```python
from build123d import *

# Parameters (mm, degrees)
F0_W        = 50
F0_H        = 30
F1_DEPTH    = 15
F2_SIZE2    = 12
F2_SIZE     = 40
F3_C1_SIZE2 = 5
F3_C1_SIZE  = 12
F3_C2_SIZE2 = 12
F3_C2_SIZE  = 5
F5_T1_DEPTH = 35.5802298817
F5_T3_DEPTH = 52.025
F5_T5_DEPTH = 27.5
F5_T7_DEPTH = 20.5
F5_T9_DEPTH = 20.5
F6_R        = 5
F7_DEPTH    = 10
F8_R        = 2.5
F8_R_2      = 2.6409986757
F9_DEPTH    = 40
F10_R       = 3.75
F11_DEPTH   = 10
F12_SIZE    = 1


# Not quite as in the source:
# - a fillet or chamfer that OpenCascade refuses, or shapes differently, is made with other operations: its cross-section is extruded or revolved along the edge and cut away or added
# - two fillets or chamfers of one size are made in one step


with BuildPart() as f1:
    # F0 (on Top) → F1 (new body)
    with BuildSketch(Plane.XY):
        with Locations((-15, 0)):
            Rectangle(F0_W, F0_H)
    extrude(amount=F1_DEPTH)

    # F2
    f2_edges = [f1.edges().sort_by_distance(p)[0] for p in [
        (-40, 0, 15),
    ]]
    f2_side = f1.faces().sort_by_distance((-15, 0, 15))[0]
    chamfer(f2_edges, length=F2_SIZE, length2=F2_SIZE2, reference=f2_side)

    # F3: chamfer of 12 x 5 on 2 edges, made by hand

    # F3_c1
    f3_c1_edges = [f1.edges().sort_by_distance(p)[0] for p in [
        (5, 15, 15),
    ]]
    f3_c1_side = f1.faces().sort_by_distance((5, 15, 14.9))[0]
    chamfer(f3_c1_edges, length=F3_C1_SIZE, length2=F3_C1_SIZE2, reference=f3_c1_side)

    # F3_c2
    f3_c2_edges = [f1.edges().sort_by_distance(p)[0] for p in [
        (5, -15, 15),
    ]]
    f3_c2_side = f1.faces().sort_by_distance((5, -14.9, 15))[0]
    chamfer(f3_c2_edges, length=F3_C2_SIZE, length2=F3_C2_SIZE2, reference=f3_c2_side)

    # F5: fillet of radius 1.5 on 6 edges, made by hand

    # F5_s2 → F5_t1 (cut)
    with BuildSketch(Plane.XZ.offset(-17.7901149408)):
        with BuildLine():
            ThreePointArc((-38.9310218283, 3.3206934515), (-39.7034393924, 2.7793498181), (-40, 1.8839540237))
            Line((-40, 1.8839540237), (-40, 3))
            Line((-40, 3), (-38.9310218283, 3.3206934515))
        make_face()
    extrude(amount=F5_T1_DEPTH, mode=Mode.SUBTRACT)

    # F5_s4 → F5_t3 (cut)
    with BuildSketch(Plane.YZ.offset(-41.275)):
        with BuildLine():
            ThreePointArc((14.8846153846, 3.2769230769), (14.9708710135, 2.9941742027), (15, 2.7))
            Line((15, 2.7), (15, 3))
            Line((15, 3), (14.8846153846, 3.2769230769))
        make_face()
        with BuildLine():
            ThreePointArc((-14.8846153846, 3.2769230769), (-14.9708710135, 2.9941742027), (-15, 2.7))
            Line((-15, 2.7), (-15, 3))
            Line((-15, 3), (-14.8846153846, 3.2769230769))
        make_face()
    extrude(amount=F5_T3_DEPTH, mode=Mode.SUBTRACT)

    # F5_s6 → F5_t5 (cut)
    with BuildSketch(Plane.XZ.offset(-13.75)):
        with BuildLine():
            ThreePointArc((10, 13.5), (9.5606601718, 14.5606601718), (8.5, 15))
            Line((8.5, 15), (10, 15))
            Line((10, 15), (10, 13.5))
        make_face()
    extrude(amount=F5_T5_DEPTH, mode=Mode.SUBTRACT)

    # F5_s8 → F5_t7 (cut)
    with BuildSketch(Plane(origin=(0, 2.5961538462, -6.2307692308), x_dir=(1, 0, 0), z_dir=(0, -0.3846153846, 0.9230769231))):
        with BuildLine():
            ThreePointArc((10, 13.5), (9.5606601718, 14.5606601718), (8.5, 15))
            Line((8.5, 15), (10, 15))
            Line((10, 15), (10, 13.5))
        make_face()
    extrude(amount=F5_T7_DEPTH, mode=Mode.SUBTRACT)

    # F5_s10 → F5_t9 (cut)
    with BuildSketch(Plane(origin=(0, 5.2884615385, 12.6923076923), x_dir=(1, 0, 0), z_dir=(0, -0.3846153846, -0.9230769231))):
        with BuildLine():
            ThreePointArc((10, 13.5), (9.5606601718, 14.5606601718), (8.5, 15))
            Line((8.5, 15), (10, 15))
            Line((10, 15), (10, 13.5))
        make_face()
    extrude(amount=F5_T9_DEPTH, mode=Mode.SUBTRACT)

    # F6 (on face) → F7 (cut)
    with BuildSketch(Plane.YZ.offset(10)):
        with Locations((0, 7.5)):
            Circle(F6_R)
    extrude(amount=-F7_DEPTH, mode=Mode.SUBTRACT)

    # F8 (on face) → F9 (cut)
    with BuildSketch(Plane(origin=(0, 0, 0), x_dir=(1, 0, 0), z_dir=(0, 0, -1))):
        with Locations((-10, 0)):
            Circle(F8_R)
        with Locations((-25, 0)):
            Circle(F8_R_2)
    extrude(amount=-F9_DEPTH, mode=Mode.SUBTRACT)

    # F10 (on face) → F11 (cut)
    with BuildSketch(Plane.XY.offset(15)):
        with Locations((-10, 0)):
            Circle(F10_R)
        with Locations((-25, 0)):
            Circle(F10_R)
    extrude(amount=-F11_DEPTH, mode=Mode.SUBTRACT)

    # F12
    f12_edges = [f1.edges().sort_by_distance(p)[0] for p in [
        (-27.640999, 0, 5),
        (-12.5, 0, 5),
    ]]
    chamfer(f12_edges, length=F12_SIZE)


solid = f1.part
```
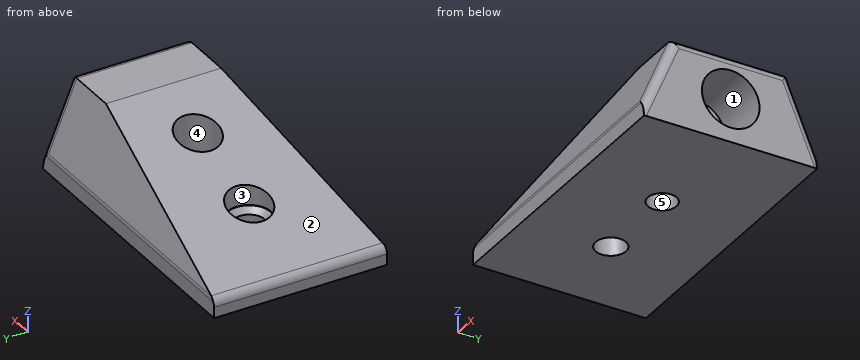
Work out the finished part from the listing and answer in its coordinate system (mm). Face numbers are marked on the shaded views. A direction names the side the tool comes from. Give positions to 0.01 mm unless a question says otherwise; leave off trailing zeros. Order: outer loops, then holes, each group sorted by start corner. A loop starts at its lowest first (then second) coordinate and runs counter-clockwise, first axis right, second up. Notation, with made-up numbers: (26, 37.5) - (41, 37.5) arc R15 cw to (41, 48.5) - close; hole circle Ø2 at (-6, 46.5). An arc over 180 degrees is marked (long way). One line per item, written item: value. Start each with the question number.
1. Each of these flat-tipped pins is pushed along its axis until it touches: pin 1 Ø2 at (x, y) = (-23, 0.5) entering from +Z; pin 2 Ø8.5 at (x, y) = (-25, 0) entering from +Z (3 decimals); pin 3 Ø8 at (x, y) = (-10, 0) entering from -Z; pin 4 Ø10 at (x, y) = (-10, 0) entering from +Z. Where does it stop, or does it pass through?
2. Consider line 1 (X direction, y = 0, z = 1.5); line 2 (Y direction, x = -10, z = 2.6); line 3 (Y direction, x = -10, z = 3.25). Determine where each line is inside the solid, lowest interval first.
3. Section C-C, the plane x = -25 is taken. Write down the section's boundary in (y, z) (3 decimals).
4. Section B-B, the plane y = 0 is taken. Count the separate pieces of the cut face and the enclosed holes in it, then the cut area to 3 significant figures.
5. For a pull along X with two mould halves and no side action, classify the marked faces 1, 2 and 3 as released by +X, released by -X, zero draft, split by the parting line, or undercut.
6. Section A-A, the plane x = -10 is taken. Write down the section's boundary in (y, z).
7. Which of the six approach directions +Z, -Z, +X, -X, +Y, -Y give full straight-line access (tool end or side, diameter ignored) to the marked faces 4 and 5?
Filled sheet:
1. pin 1: z = 4.42
1. pin 2: z = 8.775
1. pin 3: z = 0
1. pin 4: z = 13.5
2. line 1: -40 to -27.64, -22.36 to -12.5, -7.5 to 10
2. line 2: -15 to -2.5, 2.5 to 15
2. line 3: -14.9 to -2.5, 2.5 to 14.9
3. outline: (-15, 0) - (-2.641, 0) - (-2.641, 4) - (-3.641, 5) - (-3.75, 5) - (-3.75, 7.5) - (-13.125, 7.5) - (-14.885, 3.277) arc R1.5 ccw to (-15, 2.7) - close; (2.641, 0) - (15, 0) - (15, 2.7) arc R1.5 ccw to (14.885, 3.277) - (13.125, 7.5) - (3.75, 7.5) - (3.75, 5) - (3.641, 5) - (2.641, 4) - close
4. separate pieces: 3
4. enclosed holes: 0
4. area: 285 mm²
5. face 1: zero draft
5. face 2: released by -X
5. face 3: undercut
6. outline: (-15, 0) - (-2.5, 0) - (-2.5, 4) - (-3.5, 5) - (-3.75, 5) - (-3.75, 12) - (-11.25, 12) - (-14.88, 3.28) arc R1.5 ccw to (-15, 2.7) - close; (2.5, 0) - (15, 0) - (15, 2.7) arc R1.5 ccw to (14.88, 3.28) - (11.25, 12) - (3.75, 12) - (3.75, 5) - (3.5, 5) - (2.5, 4) - close
7. face 4: +Z
7. face 5: +Z, -Z
